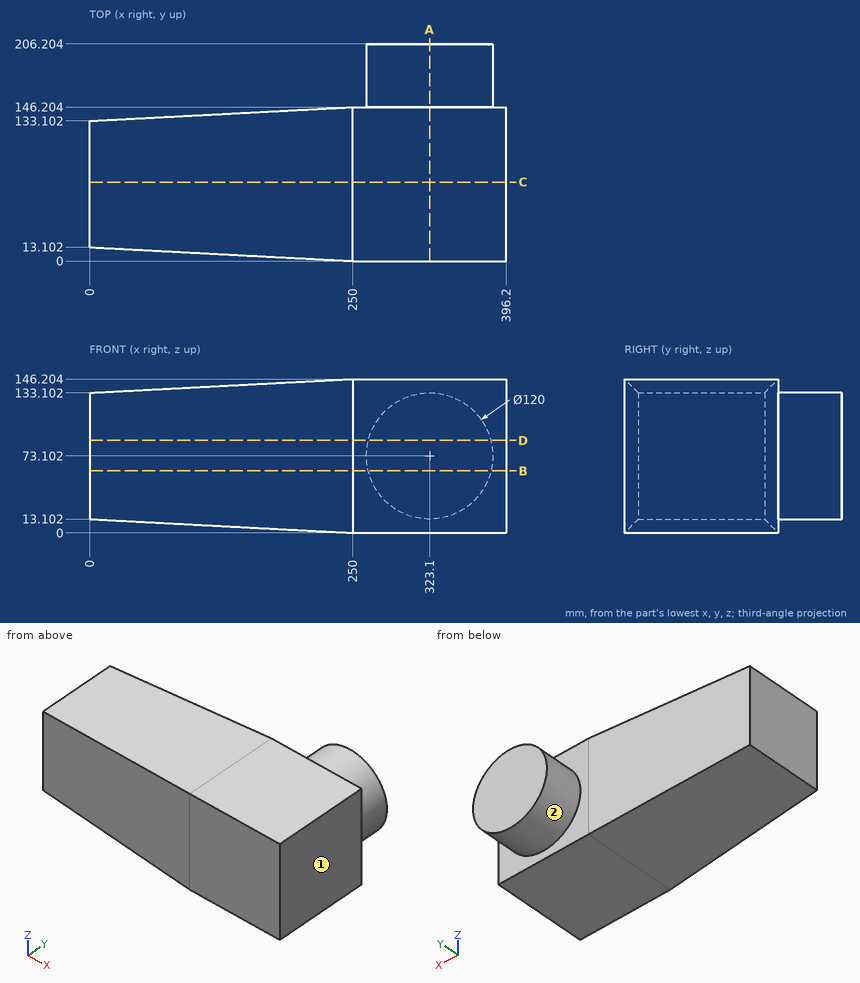
Source: three-view drawing plus pictorial views. Frame: mm from the lowest corner of the part. A direction names the side the tool comes from. Coordinates: 2 decimals unless noted, no trailing zeros. Loops run counter-clockwise (first coordinate to the right, second up) from the corner with the lowest first, then second, coordinate; pieces in that order, holes last. Notation, with made-up numbers: (66.25, -26.5) - (102.25, -26.5) arc R6 cw to (102.25, -16.5) - close; hole circle Ø8 at (-21, 10.25). An arc over 180 degrees is marked (long way). One line per question, with ' | ' between items.
1) Section A-A, the plane x = 323.1. Return loops of the section in (y, z), then the cut area to 3 significant figures.
Report:
outline: (0, 0) - (146.2, 0) - (146.2, 13.1) - (206.2, 13.1) - (206.2, 133.1) - (146.2, 133.1) - (146.2, 146.2) - (0, 146.2) - close | area: 28,600 mm²
2) First-contact query: P1, Ø5, axis at x = 79.5, y = 116.5, coming from the -Z side; P2, Ø12, axis at y = 157, z = 111.5, coming from the +X side; P3, Ø5, axis at x = 85.5, y = 50.5, coming from the +Z side; P4, Ø12, axis at y = 58.5, z = 37, coming from the -X side. Flat tips, straight axial feed; report the tip coordinate or a pass-through.
Report:
P1: stops at z = 8.8 | P2: stops at x = 373.6 | P3: stops at z = 137.71 | P4: stops at x = 0
3) Section D-D, the plane z = 88. Return loops of the section in (x, y), then the cut area to 3 significant figures.
Report:
outline: (0, 13.1) - (250, 0) - (396.2, 0) - (396.2, 146.2) - (381.22, 146.2) - (381.22, 206.2) - (264.98, 206.2) - (264.98, 146.2) - (250, 146.2) - (0, 133.1) - close | area: 61,600 mm²
4) Section C-C, the plane y = 75. Return loops of the section in (x, z), then the cut area to 3 significant figures.
Report:
outline: (0, 13.1) - (250, 0) - (396.2, 0) - (396.2, 146.2) - (250, 146.2) - (0, 133.1) - close | area: 54,700 mm²
5) Line query: line 1 along X through (y, z) = (153, 95.5); line 2 along Z through (x, y) = (244, 89.5); line 3 along Y through (x, z) = (265, 89). Output: solid intervals per line, ascending.
Report:
line 1: x = 267.44 to 378.76 | line 2: z = 0.31 to 145.89 | line 3: y = 0 to 146.2
6) Set-up query: the marked faces 1 and 2. Return all of +Z, -Z, +X, -X, +Y, -Y with unobstructed straight access to the full face (end or side cutting, diameter ignored); none if empty.
Report:
face 1: +Z, -Z, +X, +Y, -Y | face 2: +Y
7) Section B-B, the plane z = 59. Return loops of the section in (x, y).
Report:
outline: (0, 13.1) - (250, 0) - (396.2, 0) - (396.2, 146.2) - (381.42, 146.2) - (381.42, 206.2) - (264.78, 206.2) - (264.78, 146.2) - (250, 146.2) - (0, 133.1) - close
